```python
from build123d import *

# Parameters (mm, degrees)
F1_DEPTH = 10
F2_DEPTH = 4
F0_R     = 4.5
F3_DEPTH = 1.5
F4_R     = 0.5
F0_R_2   = 2.1
F5_DEPTH = 4


with BuildPart() as f1:
    # F0 (on Top) → F1 (new body)
    with BuildSketch(Plane.XY):
        with BuildLine():
            ThreePointArc((2, 6.5), (2.3717082451, 7.209430585), (2.5, 8))
            ThreePointArc((2.5, 8), (2.3717082451, 8.790569415), (2, 9.5))
            Line((2, 9.5), (-2, 9.5))
            ThreePointArc((-2, 9.5), (-2.5, 8), (-2, 6.5))
            Line((-2, 6.5), (2, 6.5))
        make_face()
    extrude(amount=F1_DEPTH)

    # F0 (on Top) → F2 (join)
    with BuildSketch(Plane.XY):
        with BuildLine():
            ThreePointArc((-2, 6.5), (0, 5.5), (2, 6.5))
            Line((2, 6.5), (-2, 6.5))
        make_face()
        with BuildLine():
            Line((-2, 9.5), (2, 9.5))
            ThreePointArc((2, 9.5), (0, 10.5), (-2, 9.5))
        make_face()
    extrude(amount=F2_DEPTH)

    # F0 (on Top) → F3 (join)
    with BuildSketch(Plane.XY):
        with Locations((0, 8)):
            Circle(F0_R)
        with BuildLine():
            ThreePointArc((2, 9.5), (2.3717082451, 8.790569415), (2.5, 8))
            ThreePointArc((2.5, 8), (2.3717082451, 7.209430585), (2, 6.5))
            ThreePointArc((2, 6.5), (0, 5.5), (-2, 6.5))
            ThreePointArc((-2, 6.5), (-2.5, 8), (-2, 9.5))
            ThreePointArc((-2, 9.5), (0, 10.5), (2, 9.5))
        make_face(mode=Mode.SUBTRACT)
    extrude(amount=F3_DEPTH)

    # F4
    f4_edges = [f1.edges().sort_by_distance(p)[0] for p in [
        (0, 9.5, 10),
        (0, 6.5, 10),
        (2.5, 8, 10),
        (-2.5, 8, 10),
    ]]
    fillet(f4_edges, radius=F4_R)

    # F0 (on Top) → F5 (join)
    with BuildSketch(Plane.XY):
        with BuildLine():
            ThreePointArc((13.5554417117, -3.5), (13.8884157477, -1.7640600948), (14, 0))
            ThreePointArc((14, 0), (13.8884157477, 1.7640600948), (13.5554417117, 3.5))
            ThreePointArc((13.5554417117, 3.5), (0, 14), (-13.5554417117, 3.5))
            ThreePointArc((-13.5554417117, 3.5), (-13.8884157477, 1.7640600948), (-14, 0))
            ThreePointArc((-14, 0), (-13.8884157477, -1.7640600948), (-13.5554417117, -3.5))
            ThreePointArc((-13.5554417117, -3.5), (0, -14), (13.5554417117, -3.5))
        make_face()
        with Locations((0, 8)):
            Circle(F0_R, mode=Mode.SUBTRACT)
        with BuildLine():
            ThreePointArc((-17.5, -3.5), (-15.0251262658, -2.4748737342), (-14, 0))
            ThreePointArc((-14, 0), (-15.0251262658, 2.4748737342), (-17.5, 3.5))
            ThreePointArc((-17.5, 3.5), (-21, 0), (-17.5, -3.5))
        make_face()
        with Locations((-17.5, 0)):
            Circle(F0_R_2, mode=Mode.SUBTRACT)
        with BuildLine():
            ThreePointArc((-14, 0), (-13.8884157477, 1.7640600948), (-13.5554417117, 3.5))
            Line((-13.5554417117, 3.5), (-17.5, 3.5))
            ThreePointArc((-17.5, 3.5), (-15.0251262658, 2.4748737342), (-14, 0))
        make_face()
        with BuildLine():
            Line((-17.5, -3.5), (-13.5554417117, -3.5))
            ThreePointArc((-13.5554417117, -3.5), (-13.8884157477, -1.7640600948), (-14, 0))
            ThreePointArc((-14, 0), (-15.0251262658, -2.4748737342), (-17.5, -3.5))
        make_face()
        with BuildLine():
            ThreePointArc((17.5, 3.5), (15.0251262658, 2.4748737342), (14, 0))
            ThreePointArc((14, 0), (15.0251262658, -2.4748737342), (17.5, -3.5))
            ThreePointArc((17.5, -3.5), (19.9748737342, -2.4748737342), (21, 0))
            ThreePointArc((21, 0), (19.9748737342, 2.4748737342), (17.5, 3.5))
        make_face()
        with Locations((17.5, 0)):
            Circle(F0_R_2, mode=Mode.SUBTRACT)
        with BuildLine():
            ThreePointArc((13.5554417117, 3.5), (13.8884157477, 1.7640600948), (14, 0))
            ThreePointArc((14, 0), (15.0251262658, 2.4748737342), (17.5, 3.5))
            Line((17.5, 3.5), (13.5554417117, 3.5))
        make_face()
        with BuildLine():
            ThreePointArc((17.5, -3.5), (15.0251262658, -2.4748737342), (14, 0))
            ThreePointArc((14, 0), (13.8884157477, -1.7640600948), (13.5554417117, -3.5))
            Line((13.5554417117, -3.5), (17.5, -3.5))
        make_face()
        with Locations((0, 8)):
            Circle(F0_R)
        with BuildLine():
            ThreePointArc((2, 9.5), (2.3717082451, 8.790569415), (2.5, 8))
            ThreePointArc((2.5, 8), (2.3717082451, 7.209430585), (2, 6.5))
            ThreePointArc((2, 6.5), (0, 5.5), (-2, 6.5))
            ThreePointArc((-2, 6.5), (-2.5, 8), (-2, 9.5))
            ThreePointArc((-2, 9.5), (0, 10.5), (2, 9.5))
        make_face(mode=Mode.SUBTRACT)
        with BuildLine():
            ThreePointArc((2, 6.5), (2.3717082451, 7.209430585), (2.5, 8))
            ThreePointArc((2.5, 8), (2.3717082451, 8.790569415), (2, 9.5))
            Line((2, 9.5), (-2, 9.5))
            ThreePointArc((-2, 9.5), (-2.5, 8), (-2, 6.5))
            Line((-2, 6.5), (2, 6.5))
        make_face()
        with BuildLine():
            ThreePointArc((-2, 6.5), (0, 5.5), (2, 6.5))
            Line((2, 6.5), (-2, 6.5))
        make_face()
        with BuildLine():
            Line((-2, 9.5), (2, 9.5))
            ThreePointArc((2, 9.5), (0, 10.5), (-2, 9.5))
        make_face()
    extrude(amount=-F5_DEPTH)


solid = f1.part
```
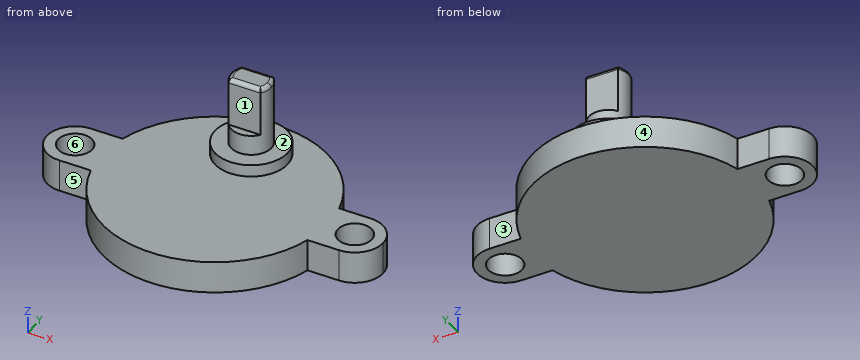
Can you work these out from the model? Positions are in its coordinate system, mm. Face numbers are marked on the shaded views. A direction names the side the tool comes from. Round coordinates to 2 decimals unless told otherwise and drop trailing zeros. Loops run counter-clockwise (first coordinate to the right, second up) from the corner with the lowest first, then second, coordinate; pieces in that order, holes last. Notation, with made-up numbers: (-6.5, 33) -> (1.5, 33) arc R22 cw to (1.5, 45) -> close; hole circle Ø3 at (62, 31.5). An arc over 180 degrees is marked (long way). One line per item, written item: value. Start each with the question number.
1. For pin 1 (10 mm diameter, centred on x = 1, y = 9.5, fed in from +Z); pin 2 (3 mm diameter, centred on x = 1, z = 7.5, fed in from -Y); pin 3 (0.8 mm diameter, centred on x = 0, y = 10, fed in from +Z); pin 4 (2.5 mm diameter, centred on x = -17.5, y = 0, fed in from -Z), each with a flat end and sliding along its axis, tell me the tip position at first contact or that it passes through.
2. If we section it at B-B, the plane y = 1.25: Write out the boundary of the cut face in (x, z).
3. If we section it at C-C, the plane y = 4.25: Write out the boundary of the cut face in (x, z).
4. If we mould it in two halves opening along X, with no side actions, what happens to the marked faces 4, 5 and 6? For each: pulls with the +X half, pulls with the -X half, needs draft (parallel to the pull), parting line crosses it, or undercut.
5. If we section it at A-A, the plane x = 18: Write out the boundary of the cut face in (y, z).
6. If I drill on probe 1 along Y at (x, z) = (-17.5, -1.85); probe 2 along Z at (x, y) = (-8.5, -11); probe 3 along Y at (x, z) = (-14, -1.25), over which ranges is the centre line in solid material (lowest first)?
7. If we section it at D-D, the plane x = 0.5: Write out the boundary of the cut face in (y, z).
8. For the marked faces 1, 2 and 3, which set-ups out of +Z, -Z, +X, -X, +Y, -Y let a thin tool reach every point of the face, with its end or its side?
Calculated:
1. pin 1: stops at z = 10
1. pin 2: stops at y = 6.5
1. pin 3: stops at z = 4
1. pin 4: passes through
2. outline: (-20.77, -4) -> (-19.19, -4) -> (-19.19, 0) -> (-20.77, 0) -> close; (-15.81, -4) -> (15.81, -4) -> (15.81, 0) -> (-15.81, 0) -> close; (19.19, -4) -> (20.77, -4) -> (20.77, 0) -> (19.19, 0) -> close
3. outline: (-13.34, -4) -> (13.34, -4) -> (13.34, 0) -> (2.49, 0) -> (2.49, 1.5) -> (-2.49, 1.5) -> (-2.49, 0) -> (-13.34, 0) -> close
4. face 4: parting line crosses it
4. face 5: needs draft
4. face 6: undercut
5. outline: (-3.46, -4) -> (-2.04, -4) -> (-2.04, 0) -> (-3.46, 0) -> close; (2.04, -4) -> (3.46, -4) -> (3.46, 0) -> (2.04, 0) -> close
6. probe 1: y = -3.5 to -2.1, 2.1 to 3.5
6. probe 2: z = -4 to 0
6. probe 3: y = -3.5 to 3.5
7. outline: (-13.99, -4) -> (13.99, -4) -> (13.99, 0) -> (12.47, 0) -> (12.47, 1.5) -> (10.45, 1.5) -> (10.45, 4) -> (9.5, 4) -> (9.5, 9.5) arc R0.5 ccw to (9, 10) -> (7, 10) arc R0.5 ccw to (6.5, 9.5) -> (6.5, 4) -> (5.55, 4) -> (5.55, 1.5) -> (3.53, 1.5) -> (3.53, 0) -> (-13.99, 0) -> close
8. face 1: +Z, +X, -X, -Y
8. face 2: +Z
8. face 3: +Z, -Z, +X, +Y
